Here's how the part is built. I have some questions about the finished solid (model axes, mm). Round coordinates to 2 decimals unless told otherwise and drop trailing zeros. Order: outer loops, then holes, each group sorted by start corner. A loop starts at its lowest first (then second) coordinate and runs counter-clockwise, first axis right, second up. Notation, with made-up numbers: (62, 88) -> (89, 88) arc R17 ccw to (89, 117) -> close; hole circle Ø5 at (2.5, 48). An arc over 180 degrees is marked (long way). One line per item, written item: value.
Autodesk Inventor part; units mm, degrees
ref_plane "YZ Plane" through (0, 0, 0) normal (1, 0, 0) x (0, 1, 0)
ref_plane "XZ Plane" through (0, 0, 0) normal (0, 1, 0) x (-1, 0, 0)
sketch "Sketch1" plane through (0, 0, 0) normal (0, 0, 1) x (1, 0, 0)
  circle A0 centre (0, 0) radius 5
  dimension "d0" = 10
extrude "Extrusion1" add sketch "Sketch1" along normal mid plane 90
fillet "Fillet1" radius 2 1 edges at (-5, 0, 45)
fillet "Fillet2" radius 2 1 edges at (-5, 0, -45)
ref_plane "Work Plane1" through (0, 0, 40) normal (0, 0, 1) x (1, 0, 0)
sketch "Sketch2" plane through (0, 0, 40) normal (0, 0, 1) x (1, 0, 0)
  circle A0 centre (0, 0) radius 3
  circle A1 centre (0, 0) radius 7.5
  dimension "d6" = 15
extrude "Extrusion2" add sketch "Sketch2" along normal blind 2.5
fillet "Fillet3" radius 1 2 edges at (-7.5, 0, 42.5) (-7.5, 0, 40)
fillet "Fillet4" radius 1 1 edges at (-5, 0, 42.5)
properties part number "panda"
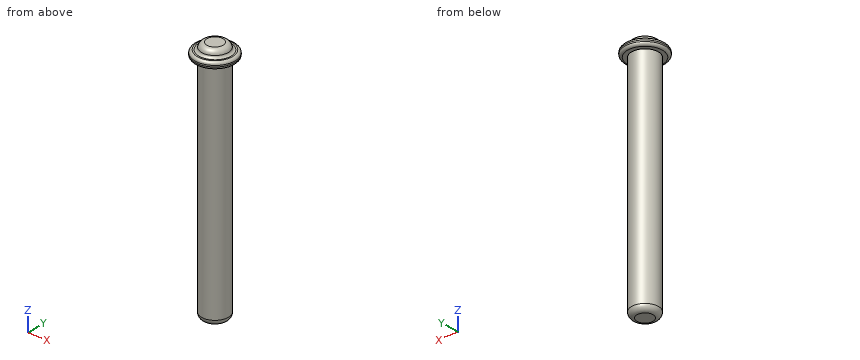
Q1. I want a section at C-C on z = -2.5. Write out the boundary of the cut face in (x, y), then the cut area to 3 significant figures.
Answers:
outline: circle Ø10 at (0, 0)
area: 78.5 mm2
Q2. For P1, Ø5, axis at y = -1, z = 8, coming from the +X side; P2, Ø4, axis at x = -3, z = 33.5, coming from the -Y side; P3, Ø1, axis at y = -5, z = -17.5, coming from the +X side, each with a flat end and sliding along its axis, tell me the tip position at first contact or that it passes through.
Answers:
P1: x = 5
P2: y = -4.9
P3: x = 2.18
Q3. I need wall thicknesses on line 1 along Z through (x, y) = (2, 6); line 2 along X through (y, z) = (-0.25, 7); line 3 along Z through (x, y) = (4.5, -5.75). Which ranges of each line are inside material? Lowest first, please.
Answers:
line 1: 40 to 42.5
line 2: -4.99 to 4.99
line 3: 40.4 to 42.1
Q4. I want a section at A-A on x = 0. Write out the boundary of the cut face in (y, z), then the cut area to 3 significant figures.
Answers:
outline: (-7.5, 41) arc R1 ccw to (-6.5, 40) -> (-5, 40) -> (-5, -43) arc R2 ccw to (-3, -45) -> (3, -45) arc R2 ccw to (5, -43) -> (5, 40) -> (6.5, 40) arc R1 ccw to (7.5, 41) -> (7.5, 41.5) arc R1 ccw to (6.5, 42.5) -> (5.96, 42.5) arc R1 cw to (4.97, 43.33) arc R2 ccw to (3, 45) -> (-3, 45) arc R2 ccw to (-4.97, 43.33) arc R1 cw to (-5.96, 42.5) -> (-6.5, 42.5) arc R1 ccw to (-7.5, 41.5) -> close
area: 909 mm2
